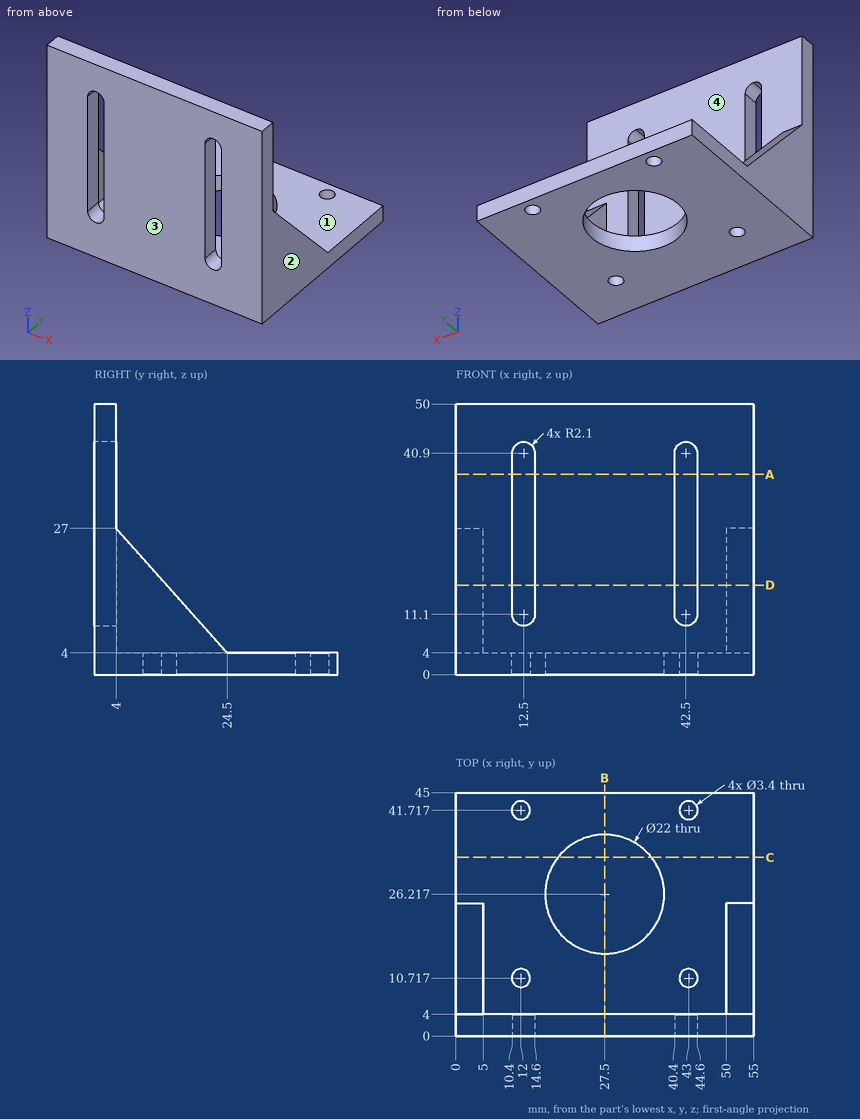
Job drawing, mm, ordinate dimensions from the low corner. One solid piece. Coordinates: 2 decimals unless noted, no trailing zeros. Order: outer loops, then holes, each group sorted by start corner. A loop starts at its lowest first (then second) coordinate and runs counter-clockwise, first axis right, second up. Notation, with made-up numbers: (-11.75, 27.25) -> (36.25, 27.25) arc R20 ccw to (36.25, 41.25) -> close; hole circle Ø9 at (36.25, 44.25). An arc over 180 degrees is marked (long way). Put each result on its own line as item: value. Start each with the question number.
(1) Band-saw the part on C-C (y = 33). Give the cut face in (x, z).
(2) Band-saw the part on B-B (x = 27.5). Give the cut face in (y, z), then the cut area to 3 significant figures.
(3) Mould opens along X. For the marked faces 1, 2, 3 and 4 say: pulls with the +X half, pulls with the -X half, needs draft (parallel to the pull), parting line crosses it, or undercut.
(4) Probe line 1 along Y through (x, z) = (43, 2.7); line 2 along X through (y, z) = (3, 30); line 3 along X through (y, z) = (15.5, 10). List the from-to ranges inside material, lowest first. Write a range as [from, to].
(5) Band-saw the part on D-D (z = 16.5). Give the cut face in (x, y).
(6) Band-saw the part on A-A (z = 37). Give the cut face in (x, y), then the cut area to 3 significant figures.
(7) Pin check, flat tips, straight feed: pin 1 Ø2 at (x, z) = (33, 16) entering from +Y; pin 2 Ø1 at (x, y) = (8.5, 6.5) entering from +Z. Stop position of each tip, or through.
Determined:
1. outline: (0, 0) -> (18.84, 0) -> (18.84, 4) -> (0, 4) -> close; (36.16, 0) -> (55, 0) -> (55, 4) -> (36.16, 4) -> close
2. outline: (0, 0) -> (15.22, 0) -> (15.22, 4) -> (4, 4) -> (4, 50) -> (0, 50) -> close; (37.22, 0) -> (45, 0) -> (45, 4) -> (37.22, 4) -> close
2. area: 276 mm²
3. face 1: undercut
3. face 2: pulls with the +X half
3. face 3: needs draft
3. face 4: undercut
4. line 1: y = [0, 9.02], [12.42, 40.02], [43.42, 45]
4. line 2: x = [0, 10.4], [14.6, 40.4], [44.6, 55]
4. line 3: x = [0, 5], [50, 55]
5. outline: (0, 0) -> (10.4, 0) -> (10.4, 4) -> (5, 4) -> (5, 13.36) -> (0, 13.36) -> close; (14.6, 0) -> (40.4, 0) -> (40.4, 4) -> (14.6, 4) -> close; (44.6, 0) -> (55, 0) -> (55, 13.36) -> (50, 13.36) -> (50, 4) -> (44.6, 4) -> close
6. outline: (0, 0) -> (10.4, 0) -> (10.4, 4) -> (0, 4) -> close; (14.6, 0) -> (40.4, 0) -> (40.4, 4) -> (14.6, 4) -> close; (44.6, 0) -> (55, 0) -> (55, 4) -> (44.6, 4) -> close
6. area: 186 mm²
7. pin 1: stops at y = 4
7. pin 2: stops at z = 4
